Part model, mm, in its own coordinate system. A direction names the side the tool comes from. Round coordinates to 2 decimals unless told otherwise and drop trailing zeros. Write each loop counter-clockwise with the first axis right and the second up, starting at its lowest first coordinate (ties: lowest second). Pieces come first, ordered by that corner, then holes. Notation, with made-up numbers: M 24,35.5 L 36,35.5 A7 ccw 36,46.5 Z; hole C -16.5,43 d7. An arc over 180 degrees is marked long. Use a Markdown table: item, result. Add a question column.
1) Drop flat-ended pins along their axis: P1, Ø1.5, axis at y = -19.5, z = 2, coming from the +X side; P2, Ø4, axis at x = -0.5, z = 9.5, coming from the -Y side; P3, Ø0.9, axis at x = 26, z = 2, coming from the +Y side. Give the stop position or say it passes through.
2) Slice it at A-A on x = -15.75. Write the cut outline in (y, z).
3) Which spindle directions (+Z, -Z, +X, -X, +Y, -Y) get a long thin tool onto all of the face, cutting with end or side? Do faces 4 (the face through (22, -7, 1)), 5 (the face through (-4, 5.1, 9.2)), 6 (the face through (-10, 24.7, 1)). Say none if no direction does.
4) Wall check: probe 1 along Y at (x, z) = (-5.75, 2.1); probe 2 along Z at (x, y) = (21.5, 0); probe 3 along Y at (x, z) = (-17, 41). Give the ranges that are in metal, low to high.
5) Slice it at C-C on z = 23.5. Write the cut outline in (x, y), plus the area to 3 significant figures.
6) Two-plate mould, pull along X, no slides. Class faces 1 (the face through (5, 3, 40.85)), 2 (the face through (12.45, -16, 2)), 3 (the face through (-3.96, 5.13, 42.25)): released by +X, released by -X, zero draft, split by the parting line, or undercut.
7) Slice it at D-D on x = -5. Give the number of separate pieces and of enclosed holes in the cut face, plus the area to 3 significant figures.
8) Slice it at B-B on y = 18. Write the cut outline in (x, z).
Autodesk Inventor part; units mm, degrees
ref_plane "Work Plane4" through (31.15, -26.2379, 8.1621) normal (1, 0, 0) x (0, 0.9775164, 0.2108593)
ref_plane "YZ Plane" through (0, 0, 0) normal (1, 0, 0) x (0, 1, 0)
ref_plane "XZ Plane" through (0, 0, 0) normal (0, 1, 0) x (-1, 0, 0)
ref_plane "Work Plane1" through (0, 0, 0) normal (0, 0, 1) x (1, 0, 0)
sketch "Sketch1" plane through (0, 0, 0) normal (0, 0, 1) x (1, 0, 0)
  circle A0 centre (-25.75, 18) radius 1.7
  circle A1 centre (4.25, 18) radius 1.7
  circle A2 centre (-15.75, 18) radius 1.7
  circle A3 centre (-5.75, 18) radius 1.7
  line L0 (-32.45, 24.7) -> (12.45, 24.7) construction
  line L1 (-32.45, 13) -> (-32.45, 24.7) construction
  line L2 (-12.45, 13) -> (-32.45, 13) construction
  line L3 (1.25, 8.4548) -> (-12.45, 13) construction
  arc A4 (5.4986, 7.8696) -> (1.25, 8.4548) centre (2.25, 0) ccw construction
  line L4 (12.45, 5) -> (5.4986, 7.8696) construction
  line L5 (12.45, 24.7) -> (12.45, 7) construction
  circle A5 centre (-25.75, -18) radius 1.7
  circle A6 centre (-15.75, -18) radius 1.7
  circle A7 centre (4.25, -18) radius 1.7
  line L6 (12.45, -24.7) -> (-32.45, -24.7) construction
  line L7 (12.45, -7) -> (12.45, -24.7) construction
  line L8 (5.4986, -7.8696) -> (12.45, -5) construction
  arc A8 (1.25, -8.4548) -> (5.4986, -7.8696) centre (2.25, 0) ccw construction
  line L9 (-12.45, -13) -> (1.25, -8.4548) construction
  line L10 (-12.45, -13) -> (-32.45, -13) construction
  line L11 (-32.45, -24.7) -> (-32.45, -13) construction
  circle A9 centre (-5.75, -18) radius 1.7
  line L12 (12.45, 24.7) -> (-32.45, 24.7)
  line L13 (-32.45, 24.7) -> (-32.45, -24.7)
  line L14 (-32.45, -24.7) -> (12.45, -24.7)
  line L15 (12.45, -24.7) -> (12.45, 24.7)
  line L16 (12.45, 5) -> (31.15, 5)
  line L17 (31.15, 5) -> (31.15, 7)
  line L18 (12.45, 7) -> (31.15, 7)
  line L19 (12.45, -7) -> (31.15, -7)
  line L20 (31.15, -7) -> (31.15, -5)
  line L21 (12.45, -5) -> (31.15, -5)
  point P0 (0, 0)
extrude "Extrusion1" add sketch "Sketch1" along normal blind 3 contours L15 L14 L13 L12
ref_plane "Work Plane2" through (-6.9588, 1.65, 41.55) normal (0, 1, 0) x (0, 0, -1)
ref_plane "Work Plane3" through (12.46, 3.65, 25.725) normal (0, 1, 0) x (0, 0, -1)
sketch "Sketch2" plane through (-6.9588, 1.65, 41.55) normal (0, 1, 0) x (0, 0, -1)
  arc A0 (29.75, -19.4088) -> (30.75, -18.4088) centre (29.75, -18.4088) ccw construction
  line L0 (30.75, -18.4088) -> (30.75, -6.9173) construction
  arc A1 (30.75, -6.9173) -> (29.8938, -5.9277) centre (29.75, -6.9173) ccw construction
  arc A2 (29.8938, 0.01) -> (29.8938, -5.9277) centre (30.325, -2.9588) ccw construction
  arc A3 (29.8938, 0.01) -> (30.75, 0.9996) centre (29.75, 0.9996) ccw construction
  line L1 (30.75, 0.9996) -> (30.75, 13.5412) construction
  arc A4 (30.75, 13.5412) -> (29.75, 14.5412) centre (29.75, 13.5412) ccw construction
  line L2 (1.9, 14.5412) -> (29.75, 14.5412) construction
  arc A5 (1.9, 14.5412) -> (0.9, 13.5412) centre (1.9, 13.5412) ccw construction
  line L3 (0.9, 13.5412) -> (0.9, 0.9996) construction
  arc A6 (0.9, 0.9996) -> (1.7563, 0.01) centre (1.9, 0.9996) ccw construction
  arc A7 (1.7563, -5.9277) -> (1.7563, 0.01) centre (1.325, -2.9588) ccw construction
  arc A8 (1.7563, -5.9277) -> (0.9, -6.9173) centre (1.9, -6.9173) ccw construction
  line L4 (0.9, -6.9173) -> (0.9, -18.4088) construction
  arc A9 (0.9, -18.4088) -> (1.9, -19.4088) centre (1.9, -18.4088) ccw construction
  line L5 (29.75, -19.4088) -> (1.9, -19.4088) construction
  line L6 (27.025, -11.9588) -> (27.025, -5.2194) construction
  line L7 (4.625, -11.9588) -> (27.025, -11.9588) construction
  line L8 (4.625, -5.2194) -> (4.625, -11.9588) construction
  arc A10 (4.625, -5.2194) -> (4.625, -0.6983) centre (1.325, -2.9588) ccw construction
  line L9 (4.625, -0.6983) -> (4.625, 11.8412) construction
  line L10 (27.025, 11.8412) -> (4.625, 11.8412) construction
  line L11 (27.025, 11.8412) -> (27.025, -0.6983) construction
  arc A11 (27.025, -0.6983) -> (27.025, -5.2194) centre (30.325, -2.9588) ccw construction
  arc A12 (33.55, -6.9286) -> (32.55, -5.9286) centre (32.55, -6.9286) ccw construction
  line L12 (32.55, -5.9286) -> (30.75, -5.9286) construction
  arc A13 (29.8938, -5.9277) -> (30.75, -5.9286) centre (30.325, -2.9588) ccw construction
  arc A14 (30.75, -6.9173) -> (29.8938, -5.9277) centre (29.75, -6.9173) ccw construction
  line L13 (30.75, -18.4088) -> (30.75, -6.9173) construction
  arc A15 (29.75, -19.4088) -> (30.75, -18.4088) centre (29.75, -18.4088) ccw construction
  line L14 (32.55, -19.4088) -> (29.75, -19.4088) construction
  arc A16 (32.55, -19.4088) -> (33.55, -18.4088) centre (32.55, -18.4088) ccw construction
  line L15 (33.55, -6.9286) -> (33.55, -18.4088) construction
  arc A17 (32.55, 0.0109) -> (33.55, 1.0109) centre (32.55, 1.0109) ccw construction
  line L16 (33.55, 13.5412) -> (33.55, 1.0109) construction
  arc A18 (33.55, 13.5412) -> (32.55, 14.5412) centre (32.55, 13.5412) ccw construction
  line L17 (29.75, 14.5412) -> (32.55, 14.5412) construction
  arc A19 (30.75, 13.5412) -> (29.75, 14.5412) centre (29.75, 13.5412) ccw construction
  line L18 (30.75, 0.9996) -> (30.75, 13.5412) construction
  arc A20 (29.8938, 0.01) -> (30.75, 0.9996) centre (29.75, 0.9996) ccw construction
  arc A21 (30.75, 0.0109) -> (29.8938, 0.01) centre (30.325, -2.9588) ccw construction
  line L19 (30.75, 0.0109) -> (32.55, 0.0109) construction
  arc A22 (-1.9, 1.0109) -> (-0.9, 0.0109) centre (-0.9, 1.0109) ccw construction
  line L20 (-0.9, 0.0109) -> (0.9, 0.0109) construction
  arc A23 (1.7563, 0.01) -> (0.9, 0.0109) centre (1.325, -2.9588) ccw construction
  arc A24 (0.9, 0.9996) -> (1.7563, 0.01) centre (1.9, 0.9996) ccw construction
  line L21 (0.9, 13.5412) -> (0.9, 0.9996) construction
  arc A25 (1.9, 14.5412) -> (0.9, 13.5412) centre (1.9, 13.5412) ccw construction
  line L22 (-0.9, 14.5412) -> (1.9, 14.5412) construction
  arc A26 (-0.9, 14.5412) -> (-1.9, 13.5412) centre (-0.9, 13.5412) ccw construction
  line L23 (-1.9, 1.0109) -> (-1.9, 13.5412) construction
  arc A27 (-0.9, -5.9286) -> (-1.9, -6.9286) centre (-0.9, -6.9286) ccw construction
  line L24 (-1.9, -18.4088) -> (-1.9, -6.9286) construction
  arc A28 (-1.9, -18.4088) -> (-0.9, -19.4088) centre (-0.9, -18.4088) ccw construction
  line L25 (1.9, -19.4088) -> (-0.9, -19.4088) construction
  arc A29 (0.9, -18.4088) -> (1.9, -19.4088) centre (1.9, -18.4088) ccw construction
  line L26 (0.9, -6.9173) -> (0.9, -18.4088) construction
  arc A30 (1.7563, -5.9277) -> (0.9, -6.9173) centre (1.9, -6.9173) ccw construction
  arc A31 (0.9, -5.9286) -> (1.7563, -5.9277) centre (1.325, -2.9588) ccw construction
  line L27 (0.9, -5.9286) -> (-0.9, -5.9286) construction
  line L28 (-1.9, -6.9286) -> (-1.9, 1.0109) construction
  arc A32 (-0.9, -5.9286) -> (-1.9, -6.9286) centre (-0.9, -6.9286) ccw construction
  line L29 (0.9, -5.9286) -> (-0.9, -5.9286) construction
  arc A33 (0.9, -5.9286) -> (0.9, 0.0109) centre (1.325, -2.9588) ccw construction
  line L30 (-0.9, 0.0109) -> (0.9, 0.0109) construction
  arc A34 (-1.9, 1.0109) -> (-0.9, 0.0109) centre (-0.9, 1.0109) ccw construction
  circle A35 centre (1.325, -2.9588) radius 1.725 construction
  line L31 (33.55, 1.0109) -> (33.55, -6.9286) construction
  arc A36 (32.55, 0.0109) -> (33.55, 1.0109) centre (32.55, 1.0109) ccw construction
  line L32 (30.75, 0.0109) -> (32.55, 0.0109) construction
  arc A37 (30.75, 0.0109) -> (30.75, -5.9286) centre (30.325, -2.9588) ccw construction
  line L33 (32.55, -5.9286) -> (30.75, -5.9286) construction
  arc A38 (33.55, -6.9286) -> (32.55, -5.9286) centre (32.55, -6.9286) ccw construction
  circle A39 centre (30.325, -2.9588) radius 1.725 construction
  line L34 (-2.3, 14.5412) -> (0.7, 14.5412)
  line L35 (0.7, -19.4088) -> (-2.3, -19.4088)
  line L36 (-2.3, -19.4088) -> (-2.3, 14.5412)
  line L37 (15.825, 14.5412) -> (15.825, -19.4088) construction
  circle A40 centre (1.325, -2.9588) radius 2.025
  line L38 (0.7, 14.5412) -> (0.7, -1.0327)
  line L39 (0.7, -4.885) -> (0.7, -19.4088)
  arc A41 (30.75, 13.5412) -> (29.75, 14.5412) centre (29.75, 13.5412) ccw construction
  line L40 (30.75, 13.5412) -> (30.75, 0.9996) construction
  arc A42 (29.8938, 0.01) -> (30.75, 0.9996) centre (29.75, 0.9996) ccw construction
  arc A43 (29.8938, 0.01) -> (29.8938, -5.9277) centre (30.325, -2.9588) ccw construction
  arc A44 (30.75, -6.9173) -> (29.8938, -5.9277) centre (29.75, -6.9173) ccw construction
  line L41 (30.75, -6.9173) -> (30.75, -18.4088) construction
  arc A45 (29.75, -19.4088) -> (30.75, -18.4088) centre (29.75, -18.4088) ccw construction
  line L42 (27.025, -5.2194) -> (27.025, -11.9588) construction
  arc A46 (27.025, -0.6983) -> (27.025, -5.2194) centre (30.325, -2.9588) ccw construction
  line L43 (27.025, -0.6983) -> (27.025, 11.8412) construction
  arc A47 (32.55, 0.0109) -> (33.55, 1.0109) centre (32.55, 1.0109) ccw construction
  line L44 (32.55, 0.0109) -> (30.75, 0.0109) construction
  arc A48 (30.75, 0.0109) -> (29.8938, 0.01) centre (30.325, -2.9588) ccw construction
  arc A49 (29.8938, 0.01) -> (30.75, 0.9996) centre (29.75, 0.9996) ccw construction
  line L45 (30.75, 13.5412) -> (30.75, 0.9996) construction
  arc A50 (30.75, 13.5412) -> (29.75, 14.5412) centre (29.75, 13.5412) ccw construction
  line L46 (32.55, 14.5412) -> (29.75, 14.5412) construction
  arc A51 (33.55, 13.5412) -> (32.55, 14.5412) centre (32.55, 13.5412) ccw construction
  line L47 (33.55, 1.0109) -> (33.55, 13.5412) construction
  arc A52 (33.55, -6.9286) -> (32.55, -5.9286) centre (32.55, -6.9286) ccw construction
  line L48 (33.55, -18.4088) -> (33.55, -6.9286) construction
  arc A53 (32.55, -19.4088) -> (33.55, -18.4088) centre (32.55, -18.4088) ccw construction
  line L49 (29.75, -19.4088) -> (32.55, -19.4088) construction
  arc A54 (29.75, -19.4088) -> (30.75, -18.4088) centre (29.75, -18.4088) ccw construction
  line L50 (30.75, -6.9173) -> (30.75, -18.4088) construction
  arc A55 (30.75, -6.9173) -> (29.8938, -5.9277) centre (29.75, -6.9173) ccw construction
  arc A56 (29.8938, -5.9277) -> (30.75, -5.9286) centre (30.325, -2.9588) ccw construction
  line L51 (30.75, -5.9286) -> (32.55, -5.9286) construction
  line L52 (33.55, -6.9286) -> (33.55, 1.0109) construction
  arc A57 (33.55, -6.9286) -> (32.55, -5.9286) centre (32.55, -6.9286) ccw construction
  line L53 (30.75, -5.9286) -> (32.55, -5.9286) construction
  arc A58 (30.75, 0.0109) -> (30.75, -5.9286) centre (30.325, -2.9588) ccw construction
  line L54 (32.55, 0.0109) -> (30.75, 0.0109) construction
  arc A59 (32.55, 0.0109) -> (33.55, 1.0109) centre (32.55, 1.0109) ccw construction
  circle A60 centre (30.325, -2.9588) radius 1.725 construction
  line L55 (33.95, 14.5412) -> (30.95, 14.5412)
  line L56 (30.95, -19.4088) -> (33.95, -19.4088)
  line L57 (33.95, -19.4088) -> (33.95, 14.5412)
  circle A61 centre (30.325, -2.9588) radius 2.025
  line L58 (30.95, 14.5412) -> (30.95, -1.0327)
  line L59 (30.95, -4.885) -> (30.95, -19.4088)
extrude "Extrusion2" add sketch "Sketch2" along normal up to surface (2 mm away) contours L34 L38 A40 L39 L35 L36 | L57 L56 L59 A61 L58 L55
sketch "Sketch3" plane through (-21.5, 3.65, 43.85) normal (0, 1, 0) x (1, 0, 0)
  line L0 (33.95, 0) -> (0, 0)
  line L1 (33.95, 36.25) -> (33.95, 33.25)
  line L2 (0, 0) -> (33.95, 0)
  line L3 (33.95, 0) -> (33.95, 36.25)
  line L4 (33.95, 36.25) -> (0, 36.25)
  line L5 (0, 36.25) -> (0, 0)
  arc A0 (15.5739, 3) -> (19.4261, 3) centre (17.5, 3.625) ccw
  arc A1 (19.4261, 33.25) -> (15.5739, 33.25) centre (17.5, 32.625) ccw
  circle A2 centre (17.5, 3.625) radius 2.025
  circle A3 centre (17.5, 32.625) radius 2.025
  circle A4 centre (17.5, 18.125) radius 5
  point P0 (21.5, 43.85)
  point P1 (33.95, 0)
  point P2 (33.95, 33.25)
  point P3 (19.4261, 33.25)
  point P4 (19.4261, 3)
  point P5 (0, 18.125)
  dimension "d15" = 10
extrude "Extrusion3" add sketch "Sketch3" along normal blind 3
sketch "Sketch4" plane through (12.45, 1.65, 7.6) normal (0, 0, -1) x (-1, 0, 0)
  line L0 (0, 0) -> (0, 5)
  line L1 (0, 0) -> (33.95, 0)
  line L2 (33.95, 0) -> (33.95, 5)
  line L3 (0, 5) -> (33.95, 5)
  point P0 (12.45, -1.65)
extrude "Extrusion4" add sketch "Sketch4" along normal up to surface (4.6 mm away)
fillet "Fillet1" radius 4 2 edges at (-4.525, 1.65, 3) (-4.525, 6.65, 3)
sketch "Sketch5" plane through (12.45, -24.7, 0) normal (1, 0, 0) x (0, 0, -1)
  line L0 (0.1, 19.7) -> (8.2, 19.7)
  line L1 (0.1, 17.7) -> (0.1, 19.7)
  line L2 (10.2, 17.7) -> (0.1, 17.7)
  line L3 (10.2, 31.7) -> (10.2, 17.7)
  line L4 (0.1, 31.7) -> (10.2, 31.7)
  line L5 (0.1, 29.7) -> (0.1, 31.7)
  line L6 (8.2, 29.7) -> (0.1, 29.7)
  line L7 (8.2, 19.7) -> (8.2, 29.7)
  line L8 (-43.85, 26.35) -> (-43.85, 31.35)
  line L9 (-43.85, 26.35) -> (-40.85, 26.35)
  line L10 (-40.85, 26.35) -> (-40.85, 28.35)
  line L11 (-40.85, 28.35) -> (-10.6, 28.35)
  line L12 (-10.6, 26.35) -> (-10.6, 28.35)
  line L13 (-10.6, 26.35) -> (-7, 26.35)
  arc A0 (-3, 22.35) -> (-7, 26.35) centre (-7, 22.35) ccw
  line L14 (-3, 0) -> (-3, 22.35)
  line L15 (0, 0) -> (-3, 0)
  line L16 (0, 0) -> (0, 49.4)
  line L17 (0, 49.4) -> (-3, 49.4)
  line L18 (-3, 35.35) -> (-3, 49.4)
  arc A1 (-7, 31.35) -> (-3, 35.35) centre (-7, 35.35) ccw
  line L19 (-43.85, 31.35) -> (-7, 31.35)
  line L20 (-3, 22.35) -> (-3, 35.35)
  line L21 (-3, 31.7) -> (0, 31.7)
  line L22 (0, 31.7) -> (0, 17.7)
  line L23 (0, 17.7) -> (-3, 17.7)
  line L24 (-3, 17.7) -> (-3, 31.7)
  line L25 (0, 0) -> (0, 49.4)
  point P0 (0, 24.7)
  point P1 (0, 31.7)
ref_plane "Work Plane4" through (31.15, -26.2379, 8.1621) normal (1, 0, 0) x (0, 0.9775164, 0.2108593)
extrude "Extrusion5" add sketch "Sketch5" along normal up to surface (18.7 mm away) contours L21 L16 L23 L14 L20
properties part number "body cover"
Entries:
| question | item | result |
|---|---|---|
| 1 | P1 | stops at x = 12.45 |
| 1 | P2 | stops at y = 1.65 |
| 1 | P3 | stops at y = 7 |
| 2 | outline | M -24.7,0 L -19.7,0 L -19.7,3 L -24.7,3 Z; M -16.3,0 L 16.3,0 L 16.3,3 L 10.65,3 A4 cw 6.65,7 L 6.65,43.85 L 1.65,43.85 L 1.65,40.85 L 3.65,40.85 L 3.65,10.6 L 1.65,10.6 L 1.65,7 A4 cw -2.35,3 L -16.3,3 Z; M 19.7,0 L 24.7,0 L 24.7,3 L 19.7,3 Z |
| 3 | face 4 | +Z, -Z, +X, -Y |
| 3 | face 5 | +Y, -Y |
| 3 | face 6 | +Z, -Z, +X, -X, +Y |
| 4 | probe 1 | y = -24.7 to -19.7, -16.3 to 16.3, 19.7 to 24.7 |
| 4 | probe 2 | z = 0 to 3 |
| 4 | probe 3 | y = 1.65 to 6.65 |
| 5 | outline | M -21.5,3.65 L -8.48,3.65 L -8.48,6.65 L -21.5,6.65 Z; M 0.48,3.65 L 12.45,3.65 L 12.45,6.65 L 0.48,6.65 Z |
| 5 | area | 75.0 mm^2 |
| 6 | face 1 | zero draft |
| 6 | face 2 | released by +X |
| 6 | face 3 | undercut |
| 7 | separate pieces | 6 |
| 7 | enclosed holes | 0 |
| 7 | area | 225 mm^2 |
| 8 | outline | M -32.45,0 L -27.45,0 L -27.45,3 L -32.45,3 Z; M -24.05,0 L -17.45,0 L -17.45,3 L -24.05,3 Z; M -14.05,0 L -7.45,0 L -7.45,3 L -14.05,3 Z; M -4.05,0 L 2.55,0 L 2.55,3 L -4.05,3 Z; M 5.95,0 L 12.45,0 L 12.45,3 L 5.95,3 Z |
